from build123d import *

# Parameters (mm, degrees)
F0_R     = 25.4
F0_R_2   = 22.225
F1_DEPTH = 1524
F2_R     = 6.35
F3_DEPTH = 25.4
F4_R     = 6.35
F5_DEPTH = 38.1


with BuildPart() as f1:
    # F0 (on Top) → F1 (new body)
    with BuildSketch(Plane.XY):
        Circle(F0_R)
        Circle(F0_R_2, mode=Mode.SUBTRACT)
    extrude(amount=F1_DEPTH)

    # F2 (on Front) → F3 (cut, symmetric)
    with BuildSketch(Plane.XZ):
        with Locations((0, 1460.5)):
            Circle(F2_R)
        with Locations((0, 63.5)):
            Circle(F2_R)
    extrude(amount=F3_DEPTH, both=True, mode=Mode.SUBTRACT)

    # F4 (on Right) → F5 (cut, symmetric)
    with BuildSketch(Plane.YZ):
        with Locations((0, 1460.5)):
            Circle(F4_R)
    extrude(amount=F5_DEPTH, both=True, mode=Mode.SUBTRACT)


solid = f1.part
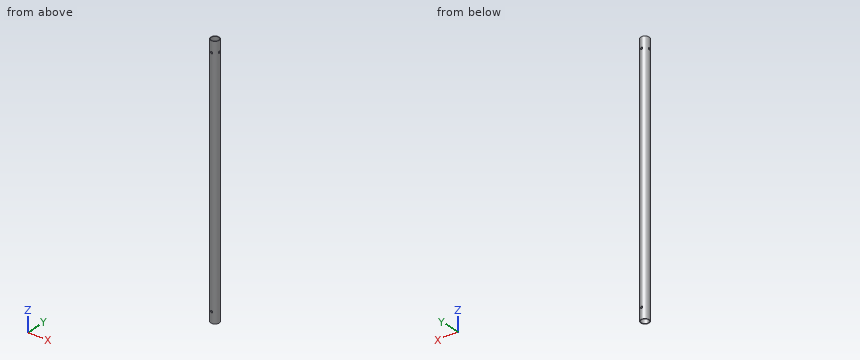
The model under review builds one solid part; all positions refer to its coordinate system, in mm. Round coordinates to 2 decimals unless told otherwise and drop trailing zeros. Write each loop counter-clockwise with the first axis right and the second up, starting at its lowest first coordinate (ties: lowest second). Pieces come first, ordered by that corner, then holes. Notation, with made-up numbers: (-39.5, 18) -> (-14.5, 18) arc R14 cw to (-14.5, 30) -> close; hole circle Ø10 at (78.5, -28). An arc over 180 degrees is marked (long way). Answer as a JSON object with one key per item and string values.
1. To check wall thickness, follow line 1 along Z through (x, y) = (23, 0); line 2 along Y through (x, z) = (0, 631) (3 decimals); line 3 along Y through (x, z) = (-2.5, 831). State the ranges of each line that lie inside material, in increasing order.
Results found:
{"line 1": "z = 0 to 1454.15, 1466.85 to 1524", "line 2": "y = -25.4 to -22.225, 22.225 to 25.4", "line 3": "y = -25.28 to -22.08, 22.08 to 25.28"}
2. Clearance check with flat-ended pins moving along their axes: pin 1 (4 mm diameter, centred on x = 7, z = 351.5, fed in from -Y); pin 2 (1 mm diameter, centred on x = -16, z = 812.5, fed in from +Y); pin 3 (5 mm diameter, centred on y = 8, z = 346, fed in from -X). State where each tip first meets the part, or that it passes through.
Results found:
{"pin 1": "stops at y = -24.9", "pin 2": "stops at y = 20.12", "pin 3": "stops at x = -24.8"}
3. We need section A-A on z = 587. State the section outline as (x, y) points (3 decimals).
Results found:
{"outline": "circle Ø50.8 at (0, 0); hole circle Ø44.45 at (0, 0)"}
